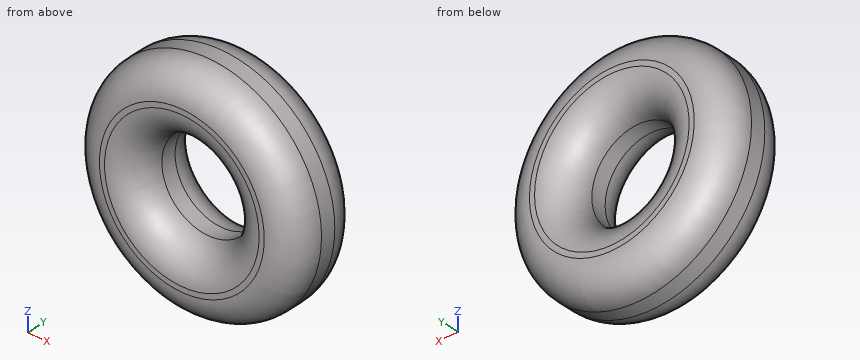
from build123d import *

# Parameters (mm, degrees)
F0_R        = 18.690948
F0_R_2      = 7.686125
F1_DEPTH    = 6.35
F2_R        = 5.08
F1_FACE_R   = 18.690948
F1_FACE_R_2 = 7.686125
F3_DEPTH    = 6.35
F4_R        = 5.08


with BuildPart() as f1:
    # F0 (on Front) → F1 (new body)
    with BuildSketch(Plane.XZ):
        Circle(F0_R)
        Circle(F0_R_2, mode=Mode.SUBTRACT)
    extrude(amount=F1_DEPTH)

    # F2
    f2_edges = [f1.edges().sort_by_distance(p)[0] for p in [
        (-18.690948, -6.35, 0),
        (-7.686125, -6.35, 0),
    ]]
    fillet(f2_edges, radius=F2_R)

    # F1_face (on face) → F3 (join)
    with BuildSketch(Plane(origin=(0, 0, 0), x_dir=(1, 0, 0), z_dir=(0, 1, 0))):
        Circle(F1_FACE_R)
        Circle(F1_FACE_R_2, mode=Mode.SUBTRACT)
    extrude(amount=F3_DEPTH)

    # F4
    f4_edges = [f1.edges().sort_by_distance(p)[0] for p in [
        (-18.690948, 6.35, 0),
        (-7.686125, 6.35, 0),
    ]]
    fillet(f4_edges, radius=F4_R)


solid = f1.part
Verification items for the finished model (mm, model axes). Round coordinates to 2 decimals unless told otherwise and drop trailing zeros. Order: outer loops, then holes, each group sorted by start corner. A loop starts at its lowest first (then second) coordinate and runs counter-clockwise, first axis right, second up.
1. Section check D-D on y = 3.25. Record the cut outline in (x, z).
Final values:
outline: circle Ø36.58 at (0, 0); hole circle Ø16.18 at (0, 0)
2. Thickness scan on L1, parallel to X at y = -0.1, z = 0; L2, parallel to Z at x = 5, y = -1. Record the ranges inside material, lowest first.
Final values:
L1: x = -18.69 to -7.69, 7.69 to 18.69
L2: z = -18.01 to -5.84, 5.84 to 18.01
3. Go/stop test with flat-tipped pins: P1, Ø6, axis at x = -9, y = 2.5, coming from the +Z side; P2, Ø1.5, axis at x = -11, y = -4, coming from the +Z side; P3, Ø6, axis at x = -0.5, y = 0.5, coming from the +Z side. Record where each tip stops, or that it passes through.
Final values:
P1: stops at z = 17.65
P2: stops at z = 14.88
P3: stops at z = 18.69
4. Section check B-B on z = 0. Record the cut outline in (x, y), then the cut area to 3 significant figures.
Final values:
outline: (-18.69, -1.27) arc R5.08 ccw to (-13.61, -6.35) - (-12.77, -6.35) arc R5.08 ccw to (-7.69, -1.27) - (-7.69, 1.27) arc R5.08 ccw to (-12.77, 6.35) - (-13.61, 6.35) arc R5.08 ccw to (-18.69, 1.27) - close; (7.69, -1.27) arc R5.08 ccw to (12.77, -6.35) - (13.61, -6.35) arc R5.08 ccw to (18.69, -1.27) - (18.69, 1.27) arc R5.08 ccw to (13.61, 6.35) - (12.77, 6.35) arc R5.08 ccw to (7.69, 1.27) - close
area: 235 mm2
5. Section check C-C on y = 0.5. Record the cut outline in (x, z).
Final values:
outline: circle Ø37.38 at (0, 0); hole circle Ø15.37 at (0, 0)
6. Section check A-A on x = 0. Record the cut outline in (y, z).
Final values:
outline: (-6.35, -13.61) arc R5.08 ccw to (-1.27, -18.69) - (1.27, -18.69) arc R5.08 ccw to (6.35, -13.61) - (6.35, -12.77) arc R5.08 ccw to (1.27, -7.69) - (-1.27, -7.69) arc R5.08 ccw to (-6.35, -12.77) - close; (-6.35, 12.77) arc R5.08 ccw to (-1.27, 7.69) - (1.27, 7.69) arc R5.08 ccw to (6.35, 12.77) - (6.35, 13.61) arc R5.08 ccw to (1.27, 18.69) - (-1.27, 18.69) arc R5.08 ccw to (-6.35, 13.61) - close
